Autodesk Inventor part; units mm, degrees
ref_plane "YZ Plane" through (0, 0, 0) normal (1, 0, 0) x (0, 1, 0)
ref_plane "XZ Plane" through (0, 0, 0) normal (0, 1, 0) x (-1, 0, 0)
ref_plane "XY Plane" through (0, 0, 0) normal (0, 0, 1) x (1, 0, 0)
sketch "Sketch3" plane through (0, 0, 0) normal (0, 1, 0) x (-1, 0, 0)
  line L0 (68.9195, -10.287) -> (-79.2178, -10.287)
  line L1 (-11.0342, -11.43) -> (-17.9938, -11.43)
  line L2 (-17.9938, -11.43) -> (-17.9938, -13.3858)
  line L3 (-11.0342, -11.43) -> (-11.0342, -13.3858)
  line L4 (-11.0342, -13.3858) -> (-13.5742, -13.3858)
  line L5 (-17.9938, -13.3858) -> (-15.4538, -13.3858)
  line L6 (-15.4538, -13.3858) -> (-15.4538, -21.59)
  line L7 (-13.5742, -13.3858) -> (-13.5742, -21.59)
  line L8 (-13.5742, -21.59) -> (-11.0342, -21.59)
  line L9 (-15.4538, -21.59) -> (-17.9938, -21.59)
  line L10 (-17.9938, -21.59) -> (-17.9938, -24.4348)
  line L11 (-11.0342, -21.59) -> (-11.0342, -24.4348)
  line L12 (-11.0342, -24.4348) -> (-17.9938, -24.4348)
  point P0 (0, 0)
  dimension "d10" = 1.143
  dimension "d11" = 6.9596
  dimension "d12" = 1.9558
  dimension "d13" = 2.54
  dimension "d14" = 2.54
  dimension "d15" = 8.2042
  dimension "d16" = 2.8448
revolve "Revolution1" add sketch "Sketch3" angle 360 about axis through (-68.9195, 0, -10.287) along (1, 0, 0)
thread "Thread1"
sketch "Sketch4" plane through (15.4538, 0, -10.287) normal (1, 0, 0) x (0, 0, -1)
  circle A0 centre (0.0087, 7.0124) radius 3.0353
  circle A1 centre (-6.6665, 2.1752) radius 3.0353
  circle A2 centre (-4.1289, -5.6681) radius 3.0353
  circle A3 centre (4.1148, -5.6783) radius 3.0353
  circle A4 centre (6.6719, 2.1587) radius 3.0353
  point P0 (-10.287, 0)
  point P1 (0, 0)
  dimension "d20" = 6.0706
  dimension "d23" = 360
extrude "Extrusion3" cut sketch "Sketch4" against normal through all
properties part number "fly wheel" material "Iron, Malleable"
Can you work these out from the model? Positions are in its coordinate system, mm. A direction names the side the tool comes from. Coordinates: 2 decimals unless noted, no trailing zeros. Loops run counter-clockwise (first coordinate to the right, second up) from the corner with the lowest first, then second, coordinate; pieces in that order, holes last. Notation, with made-up numbers: (-21, 6.5) - (-4, 6.5) arc R22 ccw to (-4, 31.5) - close; hole circle Ø2 at (7, 45.25). An arc over 180 degrees is marked (long way). Answer as a JSON object with one key per item and string values. Group by question number.
Item 1: If we section it at D-D (y = -8): List the corners of the cut face in (x, z) for me.
Item 2: If I drill on L1, parallel to Z at x = 14, y = -6; L2, parallel to Y at x = 14.5, z = -12; L3, parallel to X at y = -2.5, z = 0.25, over which ranges is the centre line in solid material (lowest first)? Write a range as from..to.
Item 3: For pin 1 (4 mm diameter, centred on x = 12.5, z = -16, fed in from +Y); pin 2 (2 mm diameter, centred on x = 17, z = -1.5, fed in from -Y); pin 3 (3 mm diameter, centred on x = 15, y = -5.5, fed in from +Z), each with a flat end and sliding along its axis, tell me the tip position at first contact or that it passes through.
Item 4: If we section it at C-C (x = 16.5): List the corners of the cut face in (y, z) for me, plus the area to 3 significant figures.
Item 5: If we section it at A-A (y = 8.75): List the corners of the cut face in (x, z) for me.
Item 6: If we section it at B-B (z = -1.75): List the corners of the cut face in (x, y) for me.
Item 7: If we mould it in two halves opening along Y, with no side actions, what happens to faces 1 (the face through (17.994, 0, -12)), 2 (the face through (13.574, -2, -13)), 3 (the face through (14.56, -8.61, 0.94)), 4 (the face through (12.322, 0.931, -13.243))? For each: released by +Y, released by -Y, zero draft, split by the parting line, or undercut.
Item 8: On a 3-axis mill with a long thin cutter (end or side, diameter ignored), from which of +Z, -Z, +X, -X, +Y, -Y can I reach the whole of each face in a straight line? I mean faces 5 (the face through (12.29, 10.03, -15.5)), 6 (the face through (16.706, -0.931, -13.243)), 7 (the face through (11.034, 0, -12)). Say none if no direction works.
Returned:
{
 "1": {"outline": "(11.03, -21.96) - (17.99, -21.96) - (17.99, -18.27) - (15.45, -18.27) - (15.45, -16.36) - (13.57, -16.36) - (13.57, -18.27) - (11.03, -18.27) - close; (11.03, -2.3) - (13.57, -2.3) - (13.57, -4.22) - (15.45, -4.22) - (15.45, -2.3) - (17.99, -2.3) - (17.99, 1.38) - (11.03, 1.38) - close; (13.57, -12.45) - (15.45, -12.45) - (15.45, -8.1) - (13.57, -8.1) - close"},
 "2": {"L1": "z = -23.1..-17.42, -11.38..-9.18, -3.14..2.53", "L2": "y = -14.04..-7.53, -3.82..4.5, 9.52..14.04", "L3": "x = 13.57..15.45"},
 "3": {"pin 1": "stops at y = 13.65", "pin 2": "stops at y = -11.81", "pin 3": "stops at z = 3.28"},
 "4": {"outline": "circle Ø28.3 at (0, -10.29); circle Ø6.2 at (0, -10.29); hole circle Ø22.61 at (0, -10.29); hole circle Ø2.29 at (0, -10.29)", "area": "254 mm²"},
 "5": {"outline": "(11.03, -21.4) - (17.99, -21.4) - (17.99, -17.44) - (15.45, -17.44) - (15.45, -12.78) - (13.57, -12.78) - (13.57, -17.44) - (11.03, -17.44) - close; (11.03, -3.13) - (13.57, -3.13) - (13.57, -7.81) - (15.45, -7.81) - (15.45, -3.13) - (17.99, -3.13) - (17.99, 0.83) - (11.03, 0.83) - close"},
 "6": {"outline": "(11.03, -11.28) - (17.99, -11.28) - (17.99, -7.41) - (15.45, -7.41) - (15.45, -0.22) - (13.57, -0.22) - (13.57, -7.41) - (11.03, -7.41) - close; (11.03, 7.41) - (13.57, 7.41) - (13.57, 4.57) - (15.45, 4.57) - (15.45, 7.41) - (17.99, 7.41) - (17.99, 11.28) - (11.03, 11.28) - close"},
 "7": {"face 1": "zero draft", "face 2": "undercut", "face 3": "split by the parting line", "face 4": "undercut"},
 "8": {"face 5": "-X", "face 6": "+X", "face 7": "+Z, -Z, -X, +Y, -Y"}
}
